```python
from build123d import *

# Parameters (mm, degrees)
SKETCH2_R           = 15
BOSS_EXTRUDE1_DEPTH = 6
BOSS_EXTRUDE2_START = 5
SKETCH3_R           = 15
BOSS_EXTRUDE2_DEPTH = 5
SKETCH4_W           = 32
SKETCH4_H           = 3
CUT_EXTRUDE1_DEPTH  = 3


with BuildPart() as part:
    # Sketch2 → Boss-Extrude1 (new, symmetric)
    with BuildSketch(Plane(origin=(0, 0, 0), x_dir=(1, 0, 0), z_dir=(0, 1, 0))):
        with Locations(Location((0, 0, 0), (0, 0, 270))):
            Circle(SKETCH2_R)
        Polygon((0, 12.846043489), (-11.125, 6.423021745), (-11.125, -6.423021745), (0, -12.846043489), (11.125, -6.423021745), (11.125, 6.423021745), align=None, mode=Mode.SUBTRACT)
    extrude(amount=BOSS_EXTRUDE1_DEPTH, both=True)

    # Sketch3 → Boss-Extrude2 (add)
    with BuildSketch(Plane(origin=(0, 6, 0), x_dir=(1, 0, 0), z_dir=(0, 1, 0)).offset(BOSS_EXTRUDE2_START)):
        with Locations(Location((0, 0, 0), (0, 0, 270))):
            Circle(SKETCH3_R)
    extrude(amount=-BOSS_EXTRUDE2_DEPTH)

    # Sketch4 → Cut-Extrude1 (cut)
    with BuildSketch(Plane(origin=(0, 11, 0), x_dir=(1, 0, 0), z_dir=(0, 1, 0))):
        Rectangle(SKETCH4_W, SKETCH4_H)
    extrude(amount=-CUT_EXTRUDE1_DEPTH, mode=Mode.SUBTRACT)


solid = part.part
```
The listing builds one solid part. Answer for the finished solid, in the listing's coordinates (mm). A direction names the side the tool comes from. Give positions to 0.01 mm unless a question says otherwise; leave off trailing zeros. Order: outer loops, then holes, each group sorted by start corner. A loop starts at its lowest first (then second) coordinate and runs counter-clockwise, first axis right, second up. Notation, with made-up numbers: M -27,-31.75 L 4,-31.75 A17 ccw 4,-13.75 Z; hole C 17,88 d10. An arc over 180 degrees is marked long. Put each result on its own line as item: value. Start each with the question number.
Item 1: The part is cut by section C-C, the plane x = 4.75. Determine the outline of the cut face in (y, z).
Item 2: Flat-ended cylindrical pins translate along their axes: P1, Ø1.5, axis at x = 4, z = 0.5, coming from the +Y side; P2, Ø1.5, axis at x = -7, y = 9, coming from the +Z side; P3, Ø6, axis at y = 5.5, z = 10, coming from the -X side. Find the tip coordinate at first contact, or state that the pin passes through.
Item 3: Find the intervals of material crossed by line 1 along X through (y, z) = (4, 0) (3 decimals); line 2 along X through (y, z) = (-1.25, 6.5); line 3 along Y through (x, z) = (1.5, -0.5), in increasing order.
Item 4: The part is cut by section D-D, the plane x = -12.75. Determine the outline of the cut face in (y, z), and give its area (3 significant figures).
Item 5: The part is cut by section B-B, the plane y = -4.5. Determine the outline of the cut face in (x, z) (3 decimals).
Item 6: Which of the six approach directions +Z, -Z, +X, -X, +Y, -Y give full straight-line access (tool end or side, diameter ignored) to faces 1 (the face through (5.48, 0.08, 9.68)), 2 (the face through (0, 11, 7)), 3 (the face through (0, 10, -1.5))?
Item 7: For a pull along Z with two mould halves and no side action, classify faces 4 (the face through (0, 11, -7)), 5 (the face through (0, 10, 1.5)), 6 (the face through (0.66, 2.619, -14.985)) as +Z half, -Z half, draft (parallel to the pull), parting line (faces both ways), or undercut.
Item 8: The part is cut by section A-A, the plane z = 0. Determine the outline of the cut face in (x, y) (3 decimals).
Answer key:
1. outline: M -6,-14.23 L 11,-14.23 L 11,-1.5 L 8,-1.5 L 8,1.5 L 11,1.5 L 11,14.23 L -6,14.23 L -6,10.1 L 6,10.1 L 6,-10.1 L -6,-10.1 Z
2. P1: stops at y = 8
2. P2: stops at z = 13.64
2. P3: stops at x = -13.27
3. line 1: x = -15 to -11.125, 11.125 to 15
3. line 2: x = -13.52 to -10.99, 10.99 to 13.52
3. line 3: y = 6 to 8
4. outline: M -6,-7.9 L 11,-7.9 L 11,-1.5 L 8,-1.5 L 8,1.5 L 11,1.5 L 11,7.9 L -6,7.9 Z
4. area: 260 mm²
5. outline: C 0,0 d30; hole M -11.125,-6.423 L 0,-12.846 L 11.125,-6.423 L 11.125,6.423 L 0,12.846 L -11.125,6.423 Z
6. face 1: -Y
6. face 2: +Z, -Z, +X, -X, +Y
6. face 3: +X, -X, +Y
7. face 4: draft
7. face 5: undercut
7. face 6: parting line
8. outline: M -15,-6 L -11.125,-6 L -11.125,6 L 11.125,6 L 11.125,-6 L 15,-6 L 15,8 L -15,8 Z
